Can you work these out from the drawing? Everything is in mm from the part's minimum corner. Coordinates: 2 decimals unless noted, no trailing zeros. Write each loop counter-clockwise with the first axis right and the second up, starting at its lowest first coordinate (ties: lowest second). Pieces come first, ordered by that corner, then holes. Notation, with made-up numbers: (16.5, 30.25) -> (32.5, 30.25) arc R18 cw to (32.5, 39.25) -> close; hole circle Ø5 at (-27.75, -39). An arc over 180 degrees is marked (long way). Answer as CSV lines item,"result". Start each with the question number.
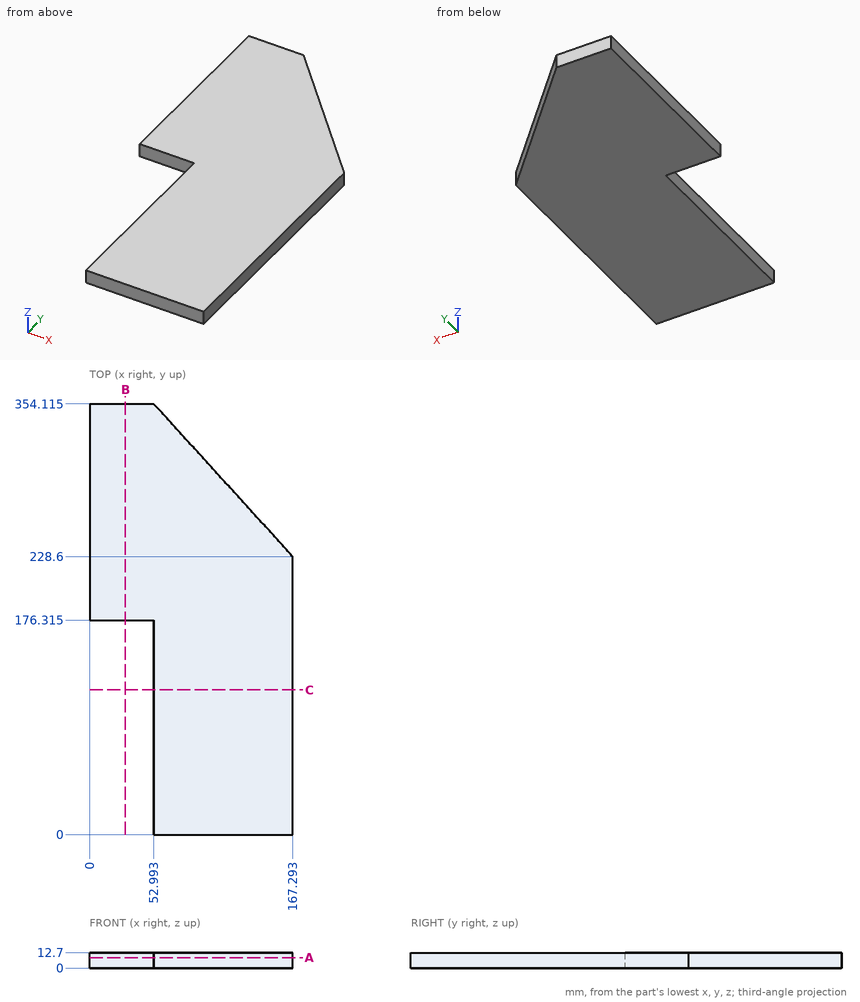
Q1. I need wall thicknesses on L1, parallel to X at y = 117, z = 5.75; L2, parallel to Y at x = 30, z = 10.75 (1 decimal); L3, parallel to Y at x = 107, z = 12.25. Which ranges of each line are inside material? Lowest first, please.
Q2. Imagine slicing it at B-B (x = 29.5). Write out the boundary of the cut face in (y, z) (1 decimal), then the cut area to 3 significant figures.
Q3. Imagine slicing it at C-C (y = 119). Write out the boundary of the cut face in (x, z).
Q4. For pin 1 (2 mm diameter, centred on y = 247.5, z = 3, fed in from +X), with a flat end and sliding along its axis, tell me the tip position at first contact or that it passes through.
Q5. Imagine slicing it at A-A (z = 8.5). Write out the boundary of the cut face in (x, y) (1 decimal).
Entries:
1,L1,"52.99 to 167.29"
1,L2,"176.3 to 354.1"
1,L3,"0 to 294.81"
2,outline,"(176.3, 0) -> (354.1, 0) -> (354.1, 12.7) -> (176.3, 12.7) -> close"
2,area,"2,260 mm2"
3,outline,"(52.99, 0) -> (167.29, 0) -> (167.29, 12.7) -> (52.99, 12.7) -> close"
4,pin 1,"x = 150.99"
5,outline,"(0, 176.3) -> (53, 176.3) -> (53, 0) -> (167.3, 0) -> (167.3, 228.6) -> (53, 354.1) -> (0, 354.1) -> close"
